Geometry: final body of the model. Coordinates: model frame, mm. A direction names the side the tool comes from. Round coordinates to 2 decimals unless told otherwise and drop trailing zeros. Order: outer loops, then holes, each group sorted by start corner. A loop starts at its lowest first (then second) coordinate and runs counter-clockwise, first axis right, second up. Notation, with made-up numbers: (-1.5, 29.5) - (32.5, 29.5) arc R29 cw to (32.5, 68.5) - close; hole circle Ø11 at (34.25, 22). An arc over 180 degrees is marked (long way). Put each result on its own line as item: value. Start each with the question number.
(1) Access query for faces 1 (the face through (100, 1.555, -6)), 2 (the face through (152, 4.476, -10)), 3 (the face through (180.733, 3.165, -5.07)). Directions: +Z, -Z, +X, -X, +Y, -Y. A direction counts if a zero-diameter tool reaches every point of the face in a straight line with its end or side. Return the directions, or none.
(2) Section B-B (y = -24). Output: boundary loops of the cut face in (x, z), and give its area (3 significant figures).
(3) Section A-A (x = 177.8). Output: boundary loops of the cut face in (y, z).
(4) Section D-D (x = 17). Output: boundary loops of the cut face in (y, z), and give its area (3 significant figures).
(5) Section C-C (x = 50.8). Output: boundary loops of the cut face in (y, z).
(6) Pin query (flat end, axial travel): P1, Ø2.5, axis at x = 151.5, z = 3, coming from the +Y side. Return the tip coordinate at first contact, or that it passes through.
(7) Material intervals for L1, parallel to Y at x = 63.5, z = 0; L2, parallel to Z at x = 165, y = -7; L3, parallel to Y at x = 49.5, z = -9, sorted ascending. Write a range as [from, to].
(8) Pull-direction query (X, two-part tool) for faces 4 (the face through (152, 4.476, 3)), 5 (the face through (100, -42.895, -6)), 6 (the face through (0, -21, 4)); classes: released by +X, released by -X, zero draft, split by the parting line, or undercut.
Autodesk Inventor part; units mm, degrees
ref_plane "YZ Plane" through (0, 0, 0) normal (1, 0, 0) x (0, 1, 0)
ref_plane "XZ Plane" through (0, 0, 0) normal (0, 1, 0) x (-1, 0, 0)
ref_plane "XY Plane" through (0, 0, 0) normal (0, 0, 1) x (1, 0, 0)
sketch "Sketch1" plane through (0, 0, 0) normal (1, 0, 0) x (0, 1, 0)
  line L0 (4.7302, 6.4139) -> (-46.0698, 6.4139)
  line L1 (-46.0698, 6.4139) -> (-46.0698, -18.9861)
  line L2 (-46.0698, -18.9861) -> (4.7302, -18.9861)
  line L3 (4.7302, -18.9861) -> (4.7302, 6.4139)
  line L4 (1.5552, 3.2389) -> (-42.8948, 3.2389)
  line L5 (-42.8948, 3.2389) -> (-42.8948, -15.8111)
  line L6 (-42.8948, -15.8111) -> (1.5552, -15.8111)
  line L7 (1.5552, -15.8111) -> (1.5552, 3.2389)
  point P0 (0, 0)
  dimension "d0" = 50.8
  dimension "d1" = 25.4
  dimension "d2" = 3.175
extrude "Extrusion1" add sketch "Sketch1" along normal blind 203.2
sketch "Sketch2" plane through (0, 4.7302, 6.4139) normal (0, 1, 0) x (1, 0, 0)
  line L0 (0, 3.175) -> (0, 22.225)
  line L1 (0, 12.7) -> (127, 12.7) construction
  line L2 (127, 12.7) -> (177.8, 12.7) construction
  circle A0 centre (177.8, 12.7) radius 3.175
  line L3 (25.4, 12.7) -> (76.2, 12.7) construction
  circle A1 centre (76.2, 12.7) radius 3.175
  point P0 (0, 6.4139)
  dimension "d30" = 50.8
  dimension "d31" = 6.35
  dimension "d32" = 50.8
  dimension "d33" = 6.35
extrude "Extrusion2" cut sketch "Sketch2" against normal blind 203.2
sketch "Sketch3" plane through (0, 4.7302, 6.4139) normal (0, 1, 0) x (1, 0, 0)
  line L0 (0, 25.4) -> (203.2, 25.4)
  line L1 (0, 22.225) -> (0, 3.175)
  circle A0 centre (66.802, 16.6589) radius 2.2987
  circle A1 centre (66.802, 3.1715) radius 2.2987
  circle A2 centre (50.8, 3.1715) radius 2.2987
  circle A3 centre (152.4, 16.6589) radius 2.2987
  circle A4 centre (152.4, 3.1715) radius 2.2987
  circle A5 centre (168.402, 3.1715) radius 2.2987
  circle A6 centre (168.402, 16.6589) radius 2.2987
  circle A7 centre (50.8, 16.6589) radius 2.2987
  point P0 (0, 6.4139)
extrude "Extrusion3" cut sketch "Sketch3" against normal blind 0.254
properties part number "Clamp Mount Aligner v2"
Checks:
1. face 1: +X, -X
1. face 2: +Y
1. face 3: +Y, -Y
2. outline: (0, -18.99) - (203.2, -18.99) - (203.2, -15.81) - (0, -15.81) - close; (0, 3.24) - (203.2, 3.24) - (203.2, 6.41) - (0, 6.41) - close
2. area: 1,290 mm²
3. outline: (-46.07, -18.99) - (4.73, -18.99) - (4.73, -9.46) - (1.56, -9.46) - (1.56, -15.81) - (-42.89, -15.81) - (-42.89, -9.46) - (-46.07, -9.46) - close; (-46.07, -3.11) - (-42.89, -3.11) - (-42.89, 3.24) - (1.56, 3.24) - (1.56, -3.11) - (4.73, -3.11) - (4.73, 6.41) - (-46.07, 6.41) - close
4. outline: (-46.07, -18.99) - (4.73, -18.99) - (4.73, 6.41) - (-46.07, 6.41) - close; hole (-42.89, -15.81) - (1.56, -15.81) - (1.56, 3.24) - (-42.89, 3.24) - close
4. area: 444 mm²
5. outline: (-46.07, -18.99) - (4.73, -18.99) - (4.73, -12.54) - (4.48, -12.54) - (4.48, -7.95) - (4.73, -7.95) - (4.73, 0.94) - (4.48, 0.94) - (4.48, 5.54) - (4.73, 5.54) - (4.73, 6.41) - (-46.07, 6.41) - close; hole (-42.89, -15.81) - (1.56, -15.81) - (1.56, 3.24) - (-42.89, 3.24) - close
6. P1: stops at y = 4.48
7. L1: y = [-46.07, -42.89], [1.56, 4.73]
7. L2: z = [-18.99, -15.81], [3.24, 6.41]
7. L3: y = [-46.07, -42.89], [1.56, 4.48]
8. face 4: undercut
8. face 5: zero draft
8. face 6: released by -X
